from build123d import *

# Parameters (mm, degrees)
BOSS_EXTRUDE1_DEPTH = 23
SHELL1_T            = -2.4
BOSS_EXTRUDE2_START = 23
SKETCH2_R           = 3
BOSS_EXTRUDE2_DEPTH = 2
BOSS_EXTRUDE2_TAPER = 30
BOSS_EXTRUDE3_START = -23
SKETCH2_2_R         = 3
BOSS_EXTRUDE3_DEPTH = 2
BOSS_EXTRUDE3_DRAFT = -30
FILLET1_R           = 1
CUT_EXTRUDE1_DEPTH  = 1
SKETCH4_W           = 40.50345243
SKETCH4_H           = 8.465012935
CUT_EXTRUDE2_DEPTH  = 50
BOSS_EXTRUDE4_START = -13.918462
SKETCH5_R           = 6.429553597
BOSS_EXTRUDE4_DEPTH = 0.3
FILLET2_R           = 1


with BuildPart() as part:
    # Sketch1 → Boss-Extrude1 (new, symmetric)
    with BuildSketch(Plane(origin=(0, 0, 0), x_dir=(0, 0, -1), z_dir=(1, 0, 0))):
        with BuildLine():
            Line((-12.176285942, -9.526430091), (-17.5, 8.473569909))
            Line((-17.5, 8.473569909), (-0.681235958, 12.395199175))
            ThreePointArc((-0.681235958, 12.395199175), (0, 12.473569909), (0.681235958, 12.395199175))
            Line((0.681235958, 12.395199175), (17.5, 8.473569909))
            Line((17.5, 8.473569909), (12.176285942, -9.526430091))
            ThreePointArc((12.176285942, -9.526430091), (0, -14.269806816), (-12.176285942, -9.526430091))
        make_face()
    extrude(amount=BOSS_EXTRUDE1_DEPTH, both=True)

    # Shell1
    shell1_openings = [part.faces().sort_by_distance(p)[0] for p in [
        (0, 10.434384542, 9.090617979),
        (0, 12.473569909, 0),
        (0, 10.434384542, -9.090617979),
    ]]
    offset(amount=SHELL1_T, openings=shell1_openings, kind=Kind.INTERSECTION)

    # Sketch2 → Boss-Extrude2 (add)
    with BuildSketch(Plane(origin=(0, 0, 0), x_dir=(0, 0, -1), z_dir=(1, 0, 0)).offset(BOSS_EXTRUDE2_START)):
        with Locations((0, 5)):
            Circle(SKETCH2_R)
    extrude(amount=BOSS_EXTRUDE2_DEPTH, taper=BOSS_EXTRUDE2_TAPER)


with BuildPart() as boss_extrude3_tool:
    # Sketch2<2> → Boss-Extrude3 (with draft: the straight prism first)
    with BuildSketch(Plane(origin=(0, 0, 0), x_dir=(0, 0, -1), z_dir=(1, 0, 0)).offset(BOSS_EXTRUDE3_START)):
        with Locations((0, 5)):
            Circle(SKETCH2_2_R)
    extrude(amount=-BOSS_EXTRUDE3_DEPTH)
    # Boss-Extrude3: the draft: its side faces are tilted about the plane it starts from
    boss_extrude3_sides = [boss_extrude3_tool.faces().sort_by_distance(p)[0] for p in [
        (-24, 5, 3),
    ]]
    draft(boss_extrude3_sides, Plane(origin=(0, 0, 0), x_dir=(0, 0, -1), z_dir=(1, 0, 0)).offset(BOSS_EXTRUDE3_START), BOSS_EXTRUDE3_DRAFT)


with BuildPart() as part_1:
    add(part.part)

    # Boss-Extrude3: add boss_extrude3_tool
    add(boss_extrude3_tool.part)

    # Fillet1
    fillet1_edges = [part_1.edges().sort_by_distance(p)[0] for p in [
        (23, -0.526430091, 14.838142971),
        (-20.6, -11.869806816, 0),
        (-20.6, 0.417860611, -12.614658399),
        (-20.6, 0.417860611, 12.614658399),
        (20.6, -11.869806816, 0),
        (20.6, 0.417860611, -12.614658399),
        (20.6, 0.417860611, 12.614658399),
        (-23, -0.526430091, 14.838142971),
        (23, -0.526430091, -14.838142971),
        (-23, -0.526430091, -14.838142971),
    ]]
    fillet(fillet1_edges, radius=FILLET1_R)

    # Sketch3 → Cut-Extrude1 (cut)
    with BuildSketch(Plane(origin=(0, -99.309611189, -14.378157577), x_dir=(1, 0, 0), z_dir=(0, 0.28361719382763534, -0.9589375826222152))):
        Polygon((-20, -96.309611189), (-1, -103.309611189), (-20, -110.309611189), align=None)
        Polygon((20, -110.309611189), (20, -96.309611189), (1, -103.309611189), align=None)
        Polygon((-16.285714286, -96.309611189), (16.285714286, -96.309611189), (0, -102.309611189), align=None)
        Polygon((-16.285714286, -110.309611189), (16.285714286, -110.309611189), (0, -104.309611189), align=None)
    cut_extrude1 = extrude(amount=CUT_EXTRUDE1_DEPTH, mode=Mode.SUBTRACT)

    # Mirror1: Cut-Extrude1 across plane
    add(cut_extrude1.mirror(Plane.XY), mode=Mode.SUBTRACT)

    # Sketch4 → Cut-Extrude2 (cut, symmetric)
    with BuildSketch(Plane(origin=(0, 0, 0), x_dir=(0, 0, -1), z_dir=(1, 0, 0))):
        with Locations((0, -18.150968344)):
            Rectangle(SKETCH4_W, SKETCH4_H)
    extrude(amount=CUT_EXTRUDE2_DEPTH, both=True, mode=Mode.SUBTRACT)

    # Sketch5 → Boss-Extrude4 (add)
    with BuildSketch(Plane(origin=(0, 0, 0), x_dir=(1, 0, 0), z_dir=(0, 1, 0)).offset(BOSS_EXTRUDE4_START)):
        with Locations((22.552407332, 0)):
            Circle(SKETCH5_R)
        with Locations((-22.552407332, 0)):
            Circle(SKETCH5_R)
    extrude(amount=BOSS_EXTRUDE4_DEPTH)

    # Fillet2
    fillet2_edges = [part_1.edges().sort_by_distance(p)[0] for p in [
        (25, 5, 1.845299462),
        (-25, 5, 1.845299462),
    ]]
    fillet(fillet2_edges, radius=FILLET2_R)


solid = part_1.part
Input: part model. Units: mm. Frame: model coordinates. A direction names the side the tool comes from. Give positions to 0.01 mm unless a question says otherwise; leave off trailing zeros. Loops run counter-clockwise (first coordinate to the right, second up) from the corner with the lowest first, then second, coordinate; pieces in that order, holes last. Notation, with made-up numbers: M 89,2.5 L 125,2.5 A28 ccw 125,23.5 Z; hole C -36.75,7.25 d1. An arc over 180 degrees is marked long. Use one line per item in the form item = value.
1. Section query D-D, the plane x = 19. Return the cut outline in (y, z), and give its area (3 significant figures).
Numbers:
outline = M -13.92,-5.36 L -13.62,-5.36 L -13.62,-4.8 A18 ccw -9.53,-12.18 L -6.6,-13.04 L -6.32,-12.08 L 6.4,-15.84 L 6.12,-16.8 L 8.47,-17.5 L 9.02,-15.16 L -8.18,-10.07 A15.6 cw -8.18,10.07 L 9.02,15.16 L 8.47,17.5 L 6.12,16.8 L 6.4,15.84 L -6.32,12.08 L -6.6,13.04 L -9.53,12.18 A18 ccw -13.62,4.8 L -13.62,5.36 L -13.92,5.36 Z
area = 119 mm²
2. Section query A-A, the plane y = 10.5. Return the cut outline in (x, z).
Numbers:
outline = M -23,-8.81 L -20.6,-8.81 L -20.6,8.81 L -23,8.81 Z; M 20.6,-8.81 L 23,-8.81 L 23,8.81 L 20.6,8.81 Z
3. Line query: L1, parallel to X at y = 5, z = -8.5; L2, parallel to X at y = -9, z = -9.5; L3, parallel to Y at x = 23.5, z = 3.5. Output: solid intervals per line, ascending.
Numbers:
L1 = -23 to -20.6, 20.6 to 23
L2 = -23 to 23
L3 = -13.92 to -13.62
4. Pull-direction query (Z, two-part tool) for faces 4 (the face through (22.715, -1.293, -14.298)), 5 (the face through (-25, 5, 0)), 6 (the face through (-10.367, 3.207, 15.428)); classes: released by +Z, released by -Z, zero draft, split by the parting line, or undercut.
Numbers:
face_4 = released by -Z
face_5 = zero draft
face_6 = undercut
5. Section query B-B, the plane z = 0. Return the cut outline in (x, y).
Numbers:
outline = M -28.98,-13.92 L 28.98,-13.92 L 28.98,-13.62 L 23,-13.62 L 23,2 L 24.5,2.87 A1 ccw 25,3.73 L 25,6.27 A1 ccw 24.5,7.13 L 23,8 L 23,12.47 L 20.6,12.47 L 20.6,-10.87 A1 cw 19.6,-11.87 L -19.6,-11.87 A1 cw -20.6,-10.87 L -20.6,12.47 L -23,12.47 L -23,8 L -24.5,7.13 A1 ccw -25,6.27 L -25,3.73 A1 ccw -24.5,2.87 L -23,2 L -23,-13.62 L -28.98,-13.62 Z
6. First-contact query: pin 1 (13 mm diameter, centred on y = 6, z = 2, fed in from -X); pin 2 (5.5 mm diameter, centred on y = 1, z = -14, fed in from +X); pin 3 (6 mm diameter, centred on y = 8.5, z = 3, fed in from -X); pin 4 (1.5 mm diameter, centred on y = -2.5, z = -15.5, fed in from -X). Flat tips, straight axial feed; report the tip coordinate or a pass-through.
Numbers:
pin_1 = -25
pin_2 = 23
pin_3 = -24.94
pin_4 = through
7. Reachability of faces 1 (the face through (0.27, -11.87, -0.15)), 2 (the face through (25, 5, 0)), 3 (the face through (-10.367, 3.207, -15.428)) from +Z, -Z, +X, -X, +Y, -Y: full face, straight path, thin tool, end or side. Return the list, or none.
Numbers:
face_1 = +Y
face_2 = +Z, -Z, +X, +Y
face_3 = none
